Autodesk Inventor part; units mm, degrees
ref_plane "YZ Plane" through (0, 0, 0) normal (1, 0, 0) x (0, 1, 0)
ref_plane "XZ Plane" through (0, 0, 0) normal (0, 1, 0) x (-1, 0, 0)
ref_plane "XY Plane" through (0, 0, 0) normal (0, 0, 1) x (1, 0, 0)
sketch "Skizze1" plane through (0, 0, 0) normal (0, 1, 0) x (-1, 0, 0)
  circle A0 centre (0, 0) radius 12.5
  circle A1 centre (0, 0) radius 11
  dimension "d0" = 25
  dimension "d1" = 22
extrude "Extrusion1" add sketch "Skizze1" along normal blind 30
sketch "Skizze2" plane through (0, 0, 0) normal (0, -1, 0) x (1, 0, 0)
  circle A0 centre (0, 0) radius 1.75
  line L0 (0, 0) -> (0, 3.5)
  line L1 (0, 3.5) -> (2.5, 3.5)
  line L2 (2.5, 3.5) -> (-2.5, 3.5)
  line L3 (-2.5, 3.5) -> (-2.5, -11.5)
  line L4 (-2.5, -11.5) -> (2.5, -11.5)
  line L5 (2.5, -11.5) -> (2.5, 3.5)
  line L6 (2.5, 3.5) -> (-2.5, 3.5)
  line L7 (-2.5, 3.5) -> (-2.5, 11.3675)
  line L8 (-2.5, 11.3675) -> (2.5, 11.3675)
  line L9 (2.5, 11.3675) -> (2.5, 3.5)
  dimension "d7" = 3.5
  dimension "d8" = 3.5
  dimension "d9" = 2.5
  dimension "d10" = 5
  dimension "d11" = 15
extrude "Extrusion2" add sketch "Skizze2" against normal blind 1
sketch "Skizze3" plane through (0, 30, 0) normal (0, 1, 0) x (1, 0, 0)
  line L0 (-17.8957, 0) -> (-17.8957, -1.5)
  line L1 (-17.8957, -1.5) -> (13.7177, -1.5)
  line L2 (13.7177, -1.5) -> (13.7177, 1.5)
  line L3 (13.7177, 1.5) -> (-17.8957, 1.5)
  line L4 (-17.8957, 1.5) -> (-17.8957, -1.5)
  point P0 (0, 0)
  dimension "d14" = 1.5
  dimension "d15" = 3
extrude "Extrusion3" cut sketch "Skizze3" against normal up to surface (29 mm away)
sketch "Skizze4" plane through (-12.4097, 1, -1.5) normal (0, 1, 0) x (1, 0, 0)
  line L0 (0, 0) -> (1.5124, 0)
  line L1 (0, 0) -> (-0.8042, 0)
  line L2 (-0.8042, 0) -> (2.2509, 0)
  line L3 (2.2509, 0) -> (2.2509, -3)
  line L4 (2.2509, -3) -> (-0.8042, -3)
  line L5 (-0.8042, -3) -> (-0.8042, 0)
  point P0 (12.4097, -1.5)
  dimension "d18" = 3
extrude "Extrusion4" cut sketch "Skizze4" against normal through all
sketch "Skizze5" plane through (10.8972, 1, 1.5) normal (0, 1, 0) x (1, 0, 0)
  line L0 (0, 0) -> (1.5124, 0)
  line L1 (0, 0) -> (2.0703, 0)
  line L2 (2.0703, 0) -> (2.0703, 3)
  line L3 (2.0703, 3) -> (0, 3)
  line L4 (0, 3) -> (0, 0)
  point P0 (-10.8972, 1.5)
  dimension "d24" = 3
extrude "Extrusion5" cut sketch "Skizze5" against normal blind 10
properties part number "CatcherModel"
For this review, take the finished solid that the model builds, in its own axes (mm). A direction names the side the tool comes from. Coordinates: 2 decimals unless noted, no trailing zeros. Loops run counter-clockwise (first coordinate to the right, second up) from the corner with the lowest first, then second, coordinate; pieces in that order, holes last.
1. Add section D-D, the plane z = -3.75. Give the boundary of the cut face in (x, y), then the cut area to 4 significant figures.
2. Add section B-B, the plane z = 0. Give the boundary of the cut face in (x, y), then the cut area to 3 significant figures.
3. For faces 1 (the flat face through (2, 1, 0)), 2 (the cylindrical face through (-0.254, 14.79, -12.497)), 3 (the flat face through (-2.5, 0.5, 0.1)), list the 3-axis set-ups (+Z, -Z, +X, -X, +Y, -Y) from which the entire face can be reached by the end or side of a thin tool; tool diameter is ignored.
4. Add section A-A, the plane y = 20.5. Give the boundary of the cut face in (x, z), then the cut area to 3 significant figures.
5. Insertion check: P1, Ø1.7, axis at x = -11.5, y = 13, coming from the +Z side; P2, Ø2.5, axis at x = 0, z = 1.5, coming from the +Y side; P3, Ø2, axis at y = 16.5, z = -7, coming from the -X side. Each pin has a flat end and moves straight along its axis. Give the tip position at first contact, or say it passes through.
6. Mouldability with a two-part tool opening along X and no side actions: class faces 4 (the cylindrical face through (0.254, 14.79, 12.497)), 5 (the flat face through (2.5, 0.5, -0.1)), 6 (the flat face through (0.1, 30, -11.5)) as +X half, -X half, draft (parallel to the pull), parting line (faces both ways), or undercut.
7. For line 1 (Z direction, x = 0, y = 0.75); line 2 (X direction, y = 0.2, z = 0); line 3 (Y direction, x = -2.25, z = -7), list the stretches that pass through material, from the lowest coordinate up.
8. Add section C-C, the plane x = 0. Give the boundary of the cut face in (y, z), then the cut area to 4 significant figures.
Result:
1. outline: (-11.92, 0) - (-10.34, 0) - (-10.34, 30) - (-11.92, 30) - close; (-2.5, 0) - (2.5, 0) - (2.5, 1) - (-2.5, 1) - close; (10.34, 0) - (11.92, 0) - (11.92, 30) - (10.34, 30) - close
1. area: 100.0 mm2
2. outline: (-2.5, 0) - (-1.75, 0) - (-1.75, 1) - (-2.5, 1) - close; (1.75, 0) - (2.5, 0) - (2.5, 1) - (1.75, 1) - close
2. area: 1.50 mm2
3. face 1: +Y
3. face 2: -Z, +Y, -Y
3. face 3: +Y, -Y
4. outline: (-12.41, -1.5) arc R12.5 ccw to (12.41, -1.5) - (10.9, -1.5) arc R11 cw to (-10.9, -1.5) - close; (-12.41, 1.5) - (-10.9, 1.5) arc R11 cw to (10.9, 1.5) - (12.41, 1.5) arc R12.5 ccw to start
4. area: 102 mm2
5. P1: stops at z = 6.54
5. P2: stops at y = 1
5. P3: stops at x = -10.97
6. face 4: parting line
6. face 5: undercut
6. face 6: draft
7. line 1: z = -12.5 to -1.75, 1.75 to 12.5
7. line 2: x = -2.5 to -1.75, 1.75 to 2.5
7. line 3: y = 0 to 1
8. outline: (0, -12.5) - (30, -12.5) - (30, -11) - (1, -11) - (1, -1.75) - (0, -1.75) - close; (0, 1.75) - (1, 1.75) - (1, 11) - (30, 11) - (30, 12.5) - (0, 12.5) - close
8. area: 108.5 mm2
